```python
from build123d import *

# Parameters (mm, degrees)
SKETCH1_W           = 68.58
SKETCH1_H           = 43.18
BOSS_EXTRUDE1_DEPTH = 2.54
SKETCH5_R           = 2.54
BOSS_EXTRUDE2_DEPTH = 2.54
SKETCH6_W           = 68.58
SKETCH6_H           = 43.18
BOSS_EXTRUDE3_DEPTH = 12.7
SKETCH7_R           = 1.4605
BOSS_EXTRUDE4_DEPTH = 2.032
SKETCH8_W           = 7.62
SKETCH8_H           = 8.2856324
CUT_EXTRUDE1_DEPTH  = 83.46203005
SKETCH9_W           = 16.129
SKETCH9_H           = 8.382
CUT_EXTRUDE2_DEPTH  = 2.032


with BuildPart() as part:
    # Sketch1 → Boss-Extrude1 (new body)
    with BuildSketch(Plane(origin=(0, 0, 0), x_dir=(1, 0, 0), z_dir=(0, 1, 0))):
        with Locations((34.29, 21.59)):
            Rectangle(SKETCH1_W, SKETCH1_H)
    extrude(amount=BOSS_EXTRUDE1_DEPTH)

    # Sketch5 → Boss-Extrude2 (add)
    with BuildSketch(Plane(origin=(0, 2.54, 0), x_dir=(1, 0, 0), z_dir=(0, 1, 0))):
        with Locations(Location((5.715, 37.465, 0), (0, 0, 90))):
            Circle(SKETCH5_R)
        with Locations(Location((62.865, 37.465, 0), (0, 0, 90))):
            Circle(SKETCH5_R)
        with Locations(Location((5.715, 5.715, 0), (0, 0, 90))):
            Circle(SKETCH5_R)
        with Locations(Location((62.865, 5.715, 0), (0, 0, 90))):
            Circle(SKETCH5_R)
    extrude(amount=BOSS_EXTRUDE2_DEPTH)

    # Sketch6 → Boss-Extrude3 (add)
    with BuildSketch(Plane(origin=(0, 2.54, 0), x_dir=(1, 0, 0), z_dir=(0, 1, 0))):
        with Locations((34.29, 21.59)):
            Rectangle(SKETCH6_W, SKETCH6_H)
        Polygon((1.27, 42.171922196), (1.27, 1.27), (67.31, 1.27), (67.31, 42.229552983), align=None, mode=Mode.SUBTRACT)
    extrude(amount=BOSS_EXTRUDE3_DEPTH)

    # Sketch7 → Boss-Extrude4 (add)
    with BuildSketch(Plane(origin=(0, 5.08, 0), x_dir=(1, 0, 0), z_dir=(0, 1, 0))):
        with Locations(Location((5.715, 37.465, 0), (0, 0, 270))):
            Circle(SKETCH7_R)
        with Locations(Location((5.715, 5.715, 0), (0, 0, 270))):
            Circle(SKETCH7_R)
        with Locations(Location((62.865, 5.715, 0), (0, 0, 270))):
            Circle(SKETCH7_R)
        with Locations(Location((62.865, 37.465, 0), (0, 0, 270))):
            Circle(SKETCH7_R)
    extrude(amount=BOSS_EXTRUDE4_DEPTH)

    # Sketch8 → Cut-Extrude1 (cut, through all)
    with BuildSketch(Plane.XY):
        with Locations((12.446, 11.0971838)):
            Rectangle(SKETCH8_W, SKETCH8_H)
    extrude(amount=-CUT_EXTRUDE1_DEPTH, mode=Mode.SUBTRACT)

    # Sketch9 → Cut-Extrude2 (cut)
    with BuildSketch(Plane(origin=(68.58, 0, 0), x_dir=(0, 0, -1), z_dir=(1, 0, 0))):
        with Locations((16.4465, 11.049)):
            Rectangle(SKETCH9_W, SKETCH9_H)
    extrude(amount=-CUT_EXTRUDE2_DEPTH, mode=Mode.SUBTRACT)


solid = part.part
```
Verification items for the finished model (mm, model axes). A direction names the side the tool comes from. Give positions to 0.01 mm unless a question says otherwise; leave off trailing zeros. Order: outer loops, then holes, each group sorted by start corner. A loop starts at its lowest first (then second) coordinate and runs counter-clockwise, first axis right, second up. Notation, with made-up numbers: M 36.25,66.25 L 76.25,66.25 A21 ccw 76.25,71.25 Z; hole C 35,2 d1. An arc over 180 degrees is marked long. Answer in a Markdown table with one row per item. Add a question column.
Item 1: Gauge pin test, flat ends, axial feed: pin 1 (0.6 mm diameter, centred on x = 68, z = -17.5, fed in from +Y); pin 2 (5.5 mm diameter, centred on x = 63, z = -37.5, fed in from +Y); pin 3 (12.5 mm diameter, centred on x = 39, z = -18.5, fed in from +Y). Record the tip position at first contact, or that the pin passes through.
Item 2: Section check A-A, the plane y = 10.75. Enter the section's corners in (x, z) (3 decimals), and give its area (3 significant figures).
Item 3: Tool access check on faces 1 (the flat face through (34, 0, -22)), 2 (the cylindrical face through (3.197, 3.792, -5.384)), 3 (the flat face through (8.636, 11, -1)), 4 (the flat face through (68, 6.858, -16)). Record the directions out of +Z, -Z, +X, -X, +Y, -Y that give a thin tool (end or side, any length) a straight path to the whole face; none if there is none.
Item 4: Scan lines: probe 1 along Z at (x, y) = (55, 13); probe 2 along X at (y, z) = (3.75, -22.5); probe 3 along Y at (x, z) = (14, -13). Record each from-to range of solid material in increasing order. Write a range as from..to.
Item 5: Section check C-C, the plane y = 5.75. Enter the section's corners in (x, z) (1 decimal), and give its area (3 significant figures).
Item 6: Mould release check, pull along X, two halves, no side actions. Record for faces 5 (the flat face through (16.256, 11, -1)), 6 (the flat face through (0, 8, -21)), 7 (the flat face through (34, 8, -43.18)): released by +X, released by -X, zero draft, split by the parting line, or undercut.
Item 7: Section check D-D, the plane x = 55.5. Enter the section's corners in (y, z), and give its area (3 significant figures).
Item 8: Section check B-B, the plane z = -23.5. Enter the section's corners in (x, y).
Filled sheet:
| question | item | result |
|---|---|---|
| 1 | pin 1 | stops at y = 6.86 |
| 1 | pin 2 | stops at y = 7.11 |
| 1 | pin 3 | stops at y = 2.54 |
| 2 | outline | M 0,-43.18 L 8.636,-43.18 L 8.636,-42.178 L 1.27,-42.172 L 1.27,-1.27 L 8.636,-1.27 L 8.636,0 L 0,0 Z; M 16.256,-43.18 L 68.58,-43.18 L 68.58,-24.511 L 67.31,-24.511 L 67.31,-42.23 L 16.256,-42.185 Z; M 16.256,-1.27 L 67.31,-1.27 L 67.31,-8.382 L 68.58,-8.382 L 68.58,0 L 16.256,0 Z |
| 2 | area | 220 mm^2 |
| 3 | face 1 | +Z, -Z, +X, -X, -Y |
| 3 | face 2 | +Y |
| 3 | face 3 | +Z, -Z, +Y |
| 3 | face 4 | +X, +Y |
| 4 | probe 1 | z = -43.18..-42.22, -1.27..0 |
| 4 | probe 2 | x = 0..1.27, 67.31..68.58 |
| 4 | probe 3 | y = 0..2.54 |
| 5 | outline | M 0,-43.2 L 68.6,-43.2 L 68.6,0 L 0,0 Z; C 5.7,-37.5 d2.9; C 5.7,-5.7 d2.9; C 62.9,-37.5 d2.9; C 62.9,-5.7 d2.9; hole M 1.3,-42.2 L 67.3,-42.2 L 67.3,-1.3 L 1.3,-1.3 Z |
| 5 | area | 285 mm^2 |
| 6 | face 5 | undercut |
| 6 | face 6 | released by -X |
| 6 | face 7 | zero draft |
| 7 | outline | M 0,-43.18 L 15.24,-43.18 L 15.24,-42.22 L 2.54,-42.22 L 2.54,-1.27 L 15.24,-1.27 L 15.24,0 L 0,0 Z |
| 7 | area | 138 mm^2 |
| 8 | outline | M 0,0 L 68.58,0 L 68.58,6.86 L 67.31,6.86 L 67.31,2.54 L 1.27,2.54 L 1.27,15.24 L 0,15.24 Z |
